Part model, mm, in its own coordinate system. Face numbers are marked on the shaded views. A direction names the side the tool comes from. Give positions to 0.01 mm unless a question says otherwise; leave off trailing zeros. Write each loop counter-clockwise with the first axis right and the second up, starting at its lowest first coordinate (ties: lowest second). Pieces come first, ordered by that corner, then holes.
from build123d import *

# Parameters (mm, degrees)
SKETCH7_W                    = 29.6256
SKETCH7_H                    = 30
BASE_FLANGE2_DEPTH           = 0.8128
EDGE_FLANGE1_STRIP_W         = 4.7244
EDGE_FLANGE1_STRIP_H         = 0.8128
EDGE_FLANGE1_STRIP_CUT_DEPTH = 30
EDGE_FLANGE1_DEPTH           = 30
EDGE_FLANGE1_FLAT_DEPTH      = 0.8128
EDGE_FLANGE3_START           = 0.7366
EDGE_FLANGE3_DEPTH           = 55.857
EDGE_FLANGE3_START_2         = 56.1872
EDGE_FLANGE3_2_DEPTH         = 0.4064
EDGE_FLANGE3_3_DEPTH         = 55.4506
CUT_EXTRUDE1_REACH           = 93.006
SKETCH21_R                   = 4.75
SKETCH21_R_2                 = 3.25
CUT_EXTRUDE2_REACH           = 88.587


# Read off the part's stored shape, not the designer's step: Edge-Flange3
# Sheet-metal steps are written as plain solids
with BuildPart() as part:
    # Sketch7 → Base-Flange2 (new body)
    with BuildSketch(Plane.YZ):
        Rectangle(SKETCH7_W, SKETCH7_H)
    extrude(amount=-BASE_FLANGE2_DEPTH)

    # Edge-Flange1 strip (across the edge) → Edge-Flange1 strip cut (cut)
    with BuildSketch(Plane(origin=(0, 14.8128, -15), x_dir=(0, -1, 0), z_dir=(0, 0, 1))):
        with Locations((-0.8128, -0.4064)):
            Rectangle(EDGE_FLANGE1_STRIP_W, EDGE_FLANGE1_STRIP_H)
    edge_flange1_strip_cut = extrude(amount=EDGE_FLANGE1_STRIP_CUT_DEPTH, mode=Mode.SUBTRACT)

    # Edge-Flange1 bend section (across the edge) → Edge-Flange1 (add)
    with BuildSketch(Plane(origin=(0, 14.8128, -15), x_dir=(0, -1, 0), z_dir=(0, 0, 1))):
        with BuildLine():
            Line((0, 0.7366), (0.8128, 0.7366))
            ThreePointArc((0.8128, 0.7366), (1.028545145, 0.215745145), (1.5494, 0))
            Line((1.5494, 0), (1.5494, -0.8128))
            ThreePointArc((1.5494, -0.8128), (0.453808753, -0.358991247), (0, 0.7366))
        make_face()
    edge_flange1 = extrude(amount=EDGE_FLANGE1_DEPTH)

    # Edge-Flange1 profile (on flange) → Edge-Flange1 flat (add)
    with BuildSketch(Plane.ZX.offset(14.8128)):
        Polygon((-40, 56.1872), (-15, 56.1872), (-15, 0.7366), (15, 0.7366), (15, 76.1872), (-40, 76.1872), align=None)
    edge_flange1_flat = extrude(amount=-EDGE_FLANGE1_FLAT_DEPTH)

    # Edge-Flange3 outline → Edge-Flange3 (cut)
    with BuildSketch(Plane.YZ.offset(EDGE_FLANGE3_START)):
        with BuildLine():
            Line((14.8128, -15), (14.8128, -14.813707039))
            ThreePointArc((14.8128, -14.813707039), (14.218624211, -14.244121367), (14, -13.4506))
            Line((14, -13.4506), (14, -15))
            Line((14, -15), (14.8128, -15))
        make_face()
    edge_flange3 = extrude(amount=EDGE_FLANGE3_DEPTH, mode=Mode.SUBTRACT)

    # Edge-Flange3 2 outline → Edge-Flange3 2 (cut)
    with BuildSketch(Plane.YZ.offset(EDGE_FLANGE3_START_2)):
        with BuildLine():
            ThreePointArc((14, -13.4506), (14.218624211, -14.244121367), (14.8128, -14.813707039))
            Line((14.8128, -14.813707039), (14.8128, -13.0442))
            Line((14.8128, -13.0442), (14, -13.0442))
            Line((14, -13.0442), (14, -13.4506))
        make_face()
    edge_flange3_2 = extrude(amount=EDGE_FLANGE3_2_DEPTH, mode=Mode.SUBTRACT)

    # Edge-Flange3 3 outline → Edge-Flange3 3 (add)
    with BuildSketch(Plane.YZ.offset(EDGE_FLANGE3_START)):
        with BuildLine():
            Line((15.5494, -15), (29, -15))
            Line((29, -15), (29, -14.1872))
            Line((29, -14.1872), (15.5494, -14.1872))
            ThreePointArc((15.5494, -14.1872), (15.028545145, -13.971454855), (14.8128, -13.4506))
            Line((14.8128, -13.4506), (14.8128, -14.813707039))
            ThreePointArc((14.8128, -14.813707039), (15.169503755, -14.952704924), (15.5494, -15))
        make_face()
    edge_flange3_3 = extrude(amount=EDGE_FLANGE3_3_DEPTH)

    # Sketch21 → Cut-Extrude1 (cut, up to next)
    with BuildSketch(Plane(origin=(0, 14.8128, 0), x_dir=(-1, 0, 0), z_dir=(0, 1, 0)), mode=Mode.PRIVATE) as cut_extrude1_sk1:
        with Locations((-66.1872, -30.16)):
            Circle(SKETCH21_R)
    cut_extrude1_tool1 = extrude(cut_extrude1_sk1.sketch, amount=-CUT_EXTRUDE1_REACH, mode=Mode.PRIVATE) & part.part
    # Sketch21 → Cut-Extrude1 (cut, up to next)
    with BuildSketch(Plane(origin=(0, 14.8128, 0), x_dir=(-1, 0, 0), z_dir=(0, 1, 0)), mode=Mode.PRIVATE) as cut_extrude1_sk2:
        with Locations((-66.1872, -7.66)):
            Circle(SKETCH21_R_2)
    cut_extrude1_tool2 = extrude(cut_extrude1_sk2.sketch, amount=-CUT_EXTRUDE1_REACH, mode=Mode.PRIVATE) & part.part
    # Sketch21 → Cut-Extrude1 (cut, up to next)
    with BuildSketch(Plane(origin=(0, 14.8128, 0), x_dir=(-1, 0, 0), z_dir=(0, 1, 0)), mode=Mode.PRIVATE) as cut_extrude1_sk3:
        with Locations((-48.982258849, 2.34)):
            Circle(SKETCH21_R_2)
    cut_extrude1_tool3 = extrude(cut_extrude1_sk3.sketch, amount=-CUT_EXTRUDE1_REACH, mode=Mode.PRIVATE) & part.part
    # Sketch21 → Cut-Extrude1 (cut, up to next)
    with BuildSketch(Plane(origin=(0, 14.8128, 0), x_dir=(-1, 0, 0), z_dir=(0, 1, 0)), mode=Mode.PRIVATE) as cut_extrude1_sk4:
        with Locations((-29.082258849, 2.34)):
            Circle(SKETCH21_R_2)
    cut_extrude1_tool4 = extrude(cut_extrude1_sk4.sketch, amount=-CUT_EXTRUDE1_REACH, mode=Mode.PRIVATE) & part.part
    # Sketch21 → Cut-Extrude1 (cut, up to next)
    with BuildSketch(Plane(origin=(0, 14.8128, 0), x_dir=(-1, 0, 0), z_dir=(0, 1, 0)), mode=Mode.PRIVATE) as cut_extrude1_sk5:
        with Locations((-9.182258849, 2.34)):
            Circle(SKETCH21_R_2)
    cut_extrude1_tool5 = extrude(cut_extrude1_sk5.sketch, amount=-CUT_EXTRUDE1_REACH, mode=Mode.PRIVATE) & part.part
    cut_extrude1_1 = cut_extrude1_tool1.solids().sort_by_distance((66.1872, 14.8128, -30.16))[0]
    add(cut_extrude1_1, mode=Mode.SUBTRACT)
    cut_extrude1_2 = cut_extrude1_tool2.solids().sort_by_distance((66.1872, 14.8128, -7.66))[0]
    add(cut_extrude1_2, mode=Mode.SUBTRACT)
    cut_extrude1_3 = cut_extrude1_tool3.solids().sort_by_distance((48.982259, 14.8128, 2.34))[0]
    add(cut_extrude1_3, mode=Mode.SUBTRACT)
    cut_extrude1_4 = cut_extrude1_tool4.solids().sort_by_distance((29.082259, 14.8128, 2.34))[0]
    add(cut_extrude1_4, mode=Mode.SUBTRACT)
    cut_extrude1_5 = cut_extrude1_tool5.solids().sort_by_distance((9.182259, 14.8128, 2.34))[0]
    add(cut_extrude1_5, mode=Mode.SUBTRACT)
    cut_extrude1 = cut_extrude1_1 + cut_extrude1_2 + cut_extrude1_3 + cut_extrude1_4 + cut_extrude1_5  # Cut-Extrude1 as one shape, for the pattern or mirror that repeats it

    # Sketch22 → Cut-Extrude2 (cut, up to next)
    with BuildSketch(Plane.XY.offset(-14.1872), mode=Mode.PRIVATE) as cut_extrude2_sk1:
        with BuildLine():
            Line((18.4866, 27.5628), (26.4866, 27.5628))
            ThreePointArc((26.4866, 27.5628), (29.2366, 24.8128), (26.4866, 22.0628))
            Line((26.4866, 22.0628), (18.4866, 22.0628))
            ThreePointArc((18.4866, 22.0628), (15.7366, 24.8128), (18.4866, 27.5628))
        make_face()
    cut_extrude2_tool1 = extrude(cut_extrude2_sk1.sketch, amount=-CUT_EXTRUDE2_REACH, mode=Mode.PRIVATE) & part.part
    # Sketch22 → Cut-Extrude2 (cut, up to next)
    with BuildSketch(Plane.XY.offset(-14.1872), mode=Mode.PRIVATE) as cut_extrude2_sk2:
        with BuildLine():
            Line((49.9866, 27.5628), (41.9866, 27.5628))
            ThreePointArc((41.9866, 27.5628), (39.2366, 24.8128), (41.9866, 22.0628))
            Line((41.9866, 22.0628), (49.9866, 22.0628))
            ThreePointArc((49.9866, 22.0628), (52.7366, 24.8128), (49.9866, 27.5628))
        make_face()
    cut_extrude2_tool2 = extrude(cut_extrude2_sk2.sketch, amount=-CUT_EXTRUDE2_REACH, mode=Mode.PRIVATE) & part.part
    cut_extrude2_1 = cut_extrude2_tool1.solids().sort_by_distance((22.4866, 24.8128, -14.1872))[0]
    add(cut_extrude2_1, mode=Mode.SUBTRACT)
    cut_extrude2_2 = cut_extrude2_tool2.solids().sort_by_distance((45.9866, 24.8128, -14.1872))[0]
    add(cut_extrude2_2, mode=Mode.SUBTRACT)
    cut_extrude2 = cut_extrude2_1 + cut_extrude2_2  # Cut-Extrude2 as one shape, for the pattern or mirror that repeats it

    # Mirror1: Edge-Flange1 strip cut, Edge-Flange1, Edge-Flange1 flat, Edge-Flange3, Edge-Flange3 2, Edge-Flange3 3, Cut-Extrude1, Cut-Extrude2 across plane
    add(edge_flange1_strip_cut.mirror(Plane.ZX), mode=Mode.SUBTRACT)
    add(edge_flange1.mirror(Plane.ZX))
    add(edge_flange1_flat.mirror(Plane.ZX))
    add(edge_flange3.mirror(Plane.ZX), mode=Mode.SUBTRACT)
    add(edge_flange3_2.mirror(Plane.ZX), mode=Mode.SUBTRACT)
    add(edge_flange3_3.mirror(Plane.ZX))
    add(cut_extrude1.mirror(Plane.ZX), mode=Mode.SUBTRACT)
    add(cut_extrude2.mirror(Plane.ZX), mode=Mode.SUBTRACT)


solid = part.part
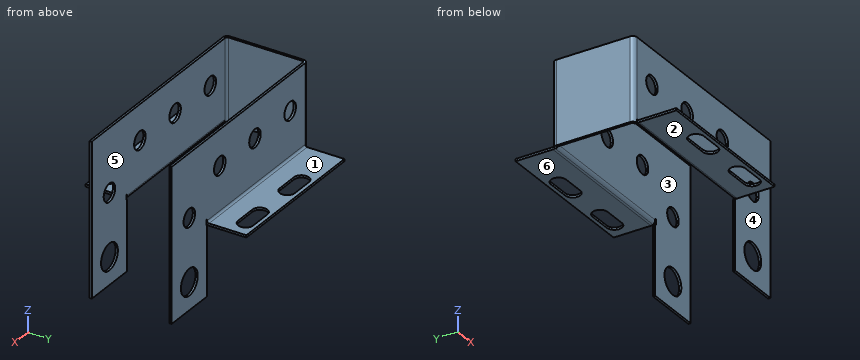
1) Saw through at A-A (x = 36). Write the cut outline in (y, z).
Check result:
outline: (-29, -15) - (-15.55, -15) arc R1.55 ccw to (-14, -13.45) - (-14, 15) - (-14.81, 15) - (-14.81, -13.45) arc R0.74 cw to (-15.55, -14.19) - (-29, -14.19) - close; (14, -13.45) arc R1.55 ccw to (15.55, -15) - (29, -15) - (29, -14.19) - (15.55, -14.19) arc R0.74 cw to (14.81, -13.45) - (14.81, 15) - (14, 15) - close
2) 3-axis set-ups, long thin cutter, end or side, ignore diameter. For the marked faces 1, 2 and 3: which of +Z, -Z, +X, -X, +Y, -Y reach the whole face in a straight line?
Check result:
face 1: +Z, +X, -X, +Y
face 2: -Z, +X, -X, +Y, -Y
face 3: +Z, -Z, +X
3) Saw through at B-B (z = -7.66). Write the cut outline in (x, y).
Check result:
outline: (-0.81, -13.26) arc R1.55 ccw to (0.74, -14.81) - (62.94, -14.81) - (62.94, -14) - (0.74, -14) arc R0.74 cw to (0, -13.26) - (0, 13.26) arc R0.74 cw to (0.74, 14) - (62.94, 14) - (62.94, 14.81) - (0.74, 14.81) arc R1.55 ccw to (-0.81, 13.26) - close; (69.44, -14.81) - (76.19, -14.81) - (76.19, -14) - (69.44, -14) - close; (69.44, 14) - (76.19, 14) - (76.19, 14.81) - (69.44, 14.81) - close
4) Saw through at C-C (z = -19). Write the cut outline in (x, y).
Check result:
outline: (56.19, -14.81) - (76.19, -14.81) - (76.19, -14) - (56.19, -14) - close; (56.19, 14) - (76.19, 14) - (76.19, 14.81) - (56.19, 14.81) - close
5) Flat gauge pins, fed straight in: P1, Ø10, axis at x = 8, y = 19, coming from the +Z side; P2, Ø5, axis at x = 57, z = -18, coming from the -Y side; P3, Ø0.8, axis at y = 19, z = -14.5, coming from the -X side; P4, Ø15, axis at x = 26, y = -22, coming from the -Z side. Where does each tip first touch, or does it go through?
Check result:
P1: stops at z = 15
P2: stops at y = -14.81
P3: stops at x = 0.74
P4: stops at z = -15
6) Mould opens along Y. For the marked faces 4, 5 and 6 say: +Y half, -Y half, draft (parallel to the pull), parting line (faces both ways), or undercut.
Check result:
face 4: -Y half
face 5: undercut
face 6: draft
7) Drill centre lines: L1, parallel to Y at x = 57, z = -3; L2, parallel to Z at x = 8, y = -16; L3, parallel to X at y = -9, z = -8. Where is each one in solid material? Low to high.
Check result:
L1: y = -14.81 to -14, 14 to 14.81
L2: z = -15 to -14.19
L3: x = -0.81 to 0
8) Saw through at D-D (z = -30.16). Write the cut outline in (x, y).
Check result:
outline: (56.19, -14.81) - (61.44, -14.81) - (61.44, -14) - (56.19, -14) - close; (56.19, 14) - (61.44, 14) - (61.44, 14.81) - (56.19, 14.81) - close; (70.94, -14.81) - (76.19, -14.81) - (76.19, -14) - (70.94, -14) - close; (70.94, 14) - (76.19, 14) - (76.19, 14.81) - (70.94, 14.81) - close
